Build history of the part. All positions in model axes, mm. Face numbers are marked on the shaded views. A direction names the side the tool comes from. Give positions to 0.01 mm unless a question says otherwise; leave off trailing zeros. Order: outer loops, then holes, each group sorted by start corner. A loop starts at its lowest first (then second) coordinate and runs counter-clockwise, first axis right, second up. Notation, with made-up numbers: (-33.75, 85.25) -> (8.25, 85.25) arc R13 ccw to (8.25, 92.25) -> close; hole circle Ø6 at (-29, 21). An arc over 180 degrees is marked (long way). One line per item, written item: value. Start each with the question number.
(1) Probe line 1 (X direction, y = 6, z = -2); line 2 (Y direction, x = -2, z = 1.75); line 3 (Z direction, x = 0, y = 21). List the from-to ranges inside material, lowest first.
(2) Saw through at A-A on z = 0. Give the cut face in (x, y) (3 decimals).
(3) Which spindle directions (+Z, -Z, +X, -X, +Y, -Y) get a long thin tool onto all of the face, cutting with end or side? Do the marked faces 1, 2, 3 and 4. Say none if no direction does.
(4) Pin check, flat tips, straight feed: pin 1 (1.5 mm diameter, centred on y = 20, z = 2.5, fed in from -X); pin 2 (1.2 mm diameter, centred on y = 12.5, z = 0, fed in from +X); pin 3 (2 mm diameter, centred on y = 11, z = 1, fed in from -X). Stop position of each tip, or through.
(5) Saw through at B-B on x = 0. Give the cut face in (y, z) (3 decimals), plus the area to 3 significant figures.
(6) Saw through at C-C on y = 21.5. Give the cut face in (x, z).
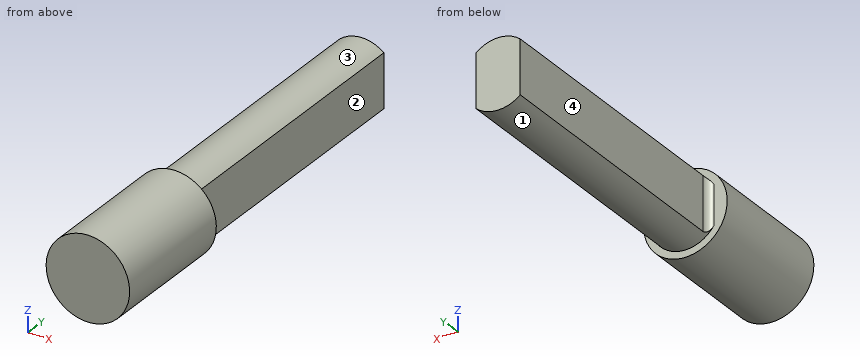
```python
from build123d import *

# Parameters (mm, degrees)
SKETCH1_R           = 3.125
BOSS_EXTRUDE1_DEPTH = 5
BOSS_EXTRUDE2_DEPTH = 21.6
FILLET1_R           = 0.5


with BuildPart() as part:
    # Sketch1 → Boss-Extrude1 (new, symmetric)
    with BuildSketch(Plane(origin=(0, 0, 0), x_dir=(1, 0, 0), z_dir=(0, 1, 0))):
        with Locations(Location((0, 0, 0), (0, 0, 270))):
            Circle(SKETCH1_R)
    extrude(amount=BOSS_EXTRUDE1_DEPTH, both=True)

    # Sketch2 → Boss-Extrude2 (add)
    with BuildSketch(Plane(origin=(0, 5, 0), x_dir=(1, 0, 0), z_dir=(0, 1, 0))):
        with BuildLine():
            Line((-1.65, -2.00935313), (-1.65, 2.00935313))
            ThreePointArc((-1.65, 2.00935313), (0, 2.6), (1.65, 2.00935313))
            Line((1.65, 2.00935313), (1.65, -2.00935313))
            ThreePointArc((1.65, -2.00935313), (0, -2.6), (-1.65, -2.00935313))
        make_face()
    extrude(amount=BOSS_EXTRUDE2_DEPTH)

    # Fillet1
    fillet1_edges = [part.edges().sort_by_distance(p)[0] for p in [
        (1.65, 5, 0),
        (-1.65, 5, 0),
    ]]
    fillet(fillet1_edges, radius=FILLET1_R)


solid = part.part
```
Results below:
1. line 1: x = -1.65 to 1.65
1. line 2: y = -5 to 5
1. line 3: z = -2.6 to 2.6
2. outline: (-3.125, -5) -> (3.125, -5) -> (3.125, 5) -> (2.15, 5) arc R0.5 cw to (1.65, 5.5) -> (1.65, 26.6) -> (-1.65, 26.6) -> (-1.65, 5.5) arc R0.5 cw to (-2.15, 5) -> (-3.125, 5) -> close
3. face 1: -Z, +Y
3. face 2: +Z, -Z, +X, +Y
3. face 3: +Z, +Y
3. face 4: +Z, -Z, -X, +Y
4. pin 1: stops at x = -1.65
4. pin 2: stops at x = 1.65
4. pin 3: stops at x = -1.65
5. outline: (-5, -3.125) -> (5, -3.125) -> (5, -2.6) -> (26.6, -2.6) -> (26.6, 2.6) -> (5, 2.6) -> (5, 3.125) -> (-5, 3.125) -> close
5. area: 175 mm²
6. outline: (-1.65, -2.01) arc R2.6 ccw to (1.65, -2.01) -> (1.65, 2.01) arc R2.6 ccw to (-1.65, 2.01) -> close
